Source: CAD feature listing. Evaluate the final solid. Frame: model axes, mm. Round coordinates to 2 decimals unless told otherwise and drop trailing zeros. Order: outer loops, then holes, each group sorted by start corner. A loop starts at its lowest first (then second) coordinate and runs counter-clockwise, first axis right, second up. Notation, with made-up numbers: M 16,-12 L 66,-12 A27 ccw 66,12 Z; hole C -36,-39.5 d10. An arc over 180 degrees is marked long. Use one line per item in the form item = value. Start each with the question number.
Q1. Contact query for flat-ended pins moving along their axis: pin 1 (1.5 mm diameter, centred on x = 2.5, y = -2.5, fed in from -Z); pin 2 (20 mm diameter, centred on y = 0, z = -38.1, fed in from +X); pin 3 (1 mm diameter, centred on x = 1.5, y = -10, fed in from +Z). Output: stop coordinate, or through.
Q2. Section C-C (z = 48). Return the cut outline in (x, y) (3 decimals).
Q3. Material intervals for probe 1 along Z at (x, y) = (2.3, -1); probe 2 along Z at (x, y) = (2.55, 4); probe 3 along Y at (x, z) = (1.2, 38.1), sorted ascending.
Q4. Section A-A (x = 0.6). Give the number of separate pieces and of enclosed holes in the cut face, plus the area to 3 significant figures.
Q5. Section D-D (y = 13). Return the cut outline in (x, z) (3 decimals), plus the area to 3 significant figures.
Q6. Section B-B (y = 0). Return the cut outline in (x, z) (1 decimal).
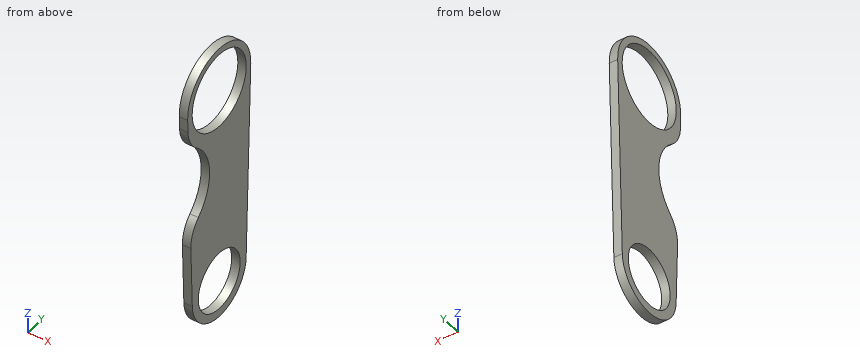
from build123d import *

# Parameters (mm, degrees)
SKETCH1_R           = 14.351
SKETCH1_R_2         = 11.1125
BOSS_EXTRUDE1_DEPTH = 3.175
SKETCH2_R           = 19.05
CUT_EXTRUDE1_DEPTH  = 58.416238601
FILLET1_R           = 12.7


with BuildPart() as part:
    # Sketch1 → Boss-Extrude1 (new body)
    with BuildSketch(Plane(origin=(0, 0, 0), x_dir=(0, 0, -1), z_dir=(1, 0, 0))):
        with BuildLine():
            Line((-37.563173646, 16.723636193), (38.558390625, 14.280144757))
            ThreePointArc((38.558390625, 14.280144757), (52.3875, 0), (38.558390625, -14.280144757))
            Line((38.558390625, -14.280144757), (-37.563173646, -16.723636193))
            ThreePointArc((-37.563173646, -16.723636193), (-54.83225, 0), (-37.563173646, 16.723636193))
        make_face()
        with Locations((-38.1, 0)):
            Circle(SKETCH1_R, mode=Mode.SUBTRACT)
        with Locations((38.1, 0)):
            Circle(SKETCH1_R_2, mode=Mode.SUBTRACT)
    extrude(amount=BOSS_EXTRUDE1_DEPTH)

    # Sketch2 → Cut-Extrude1 (cut, through all)
    with BuildSketch(Plane(origin=(3.175, 0, 0), x_dir=(0, 0, -1), z_dir=(1, 0, 0))):
        with Locations((-8.615205614, -24.13)):
            Circle(SKETCH2_R)
    extrude(amount=-CUT_EXTRUDE1_DEPTH, mode=Mode.SUBTRACT)

    # Fillet1
    fillet1_edges = [part.edges().sort_by_distance(p)[0] for p in [
        (1.5875, -15.253351608, -8.240286468),
        (1.5875, -16.352629743, 26.005289337),
    ]]
    fillet(fillet1_edges, radius=FILLET1_R)


solid = part.part
Results list:
q1.pin_1 = -52.28
q1.pin_2 = through
q1.pin_3 = 51.87
q2.outline = M 0,-13.489 L 3.175,-13.489 L 3.175,-10.389 L 0,-10.389 Z; M 0,10.389 L 3.175,10.389 L 3.175,13.489 L 0,13.489 Z
q3.probe_1 = -52.35 to -49.17, -27.03 to 23.78, 52.42 to 54.8
q3.probe_2 = -51.82 to -48.47, -27.73 to 24.32, 51.88 to 54.35
q3.probe_3 = -16.73 to -14.35, 14.35 to 16.73
q4.separate_pieces = 1
q4.enclosed_holes = 2
q4.area = 1,820 mm2
q5.outline = M 0,-44.027 L 3.175,-44.027 L 3.175,32.021 L 0,32.021 Z; M 0,44.179 L 3.175,44.179 L 3.175,48.634 L 0,48.634 Z
q5.area = 256 mm2
q6.outline = M 0,-52.4 L 3.2,-52.4 L 3.2,-49.2 L 0,-49.2 Z; M 0,-27 L 3.2,-27 L 3.2,23.7 L 0,23.7 Z; M 0,52.5 L 3.2,52.5 L 3.2,54.8 L 0,54.8 Z
